Source: CAD feature listing. Evaluate the final solid. Frame: model axes, mm. Give positions to 0.01 mm unless a question says otherwise; leave off trailing zeros. Write each loop counter-clockwise with the first axis right and the second up, starting at its lowest first coordinate (ties: lowest second). Pieces come first, ordered by that corner, then holes. Notation, with made-up numbers: (83.5, -5.75) - (122.5, -5.75) arc R14 ccw to (122.5, 1.25) - close; hole circle Ø1 at (22.5, 12.5). An arc over 180 degrees is marked (long way). One line per question, with ' | ' between items. Start each with the question number.
(1) Section C-C, the plane x = 8. Return loops of the section in (y, z).
(2) Section A-A, the plane x = 16.5. Return loops of the section in (y, z).
(3) Section B-B, the plane y = 18.5. Return loops of the section in (x, z), plus the area to 3 significant figures.
(4) Ray query, line 1 (Z direction, x = -25, y = 0.5). Return the intervals inside material, ascending. Write a range as [from, to].
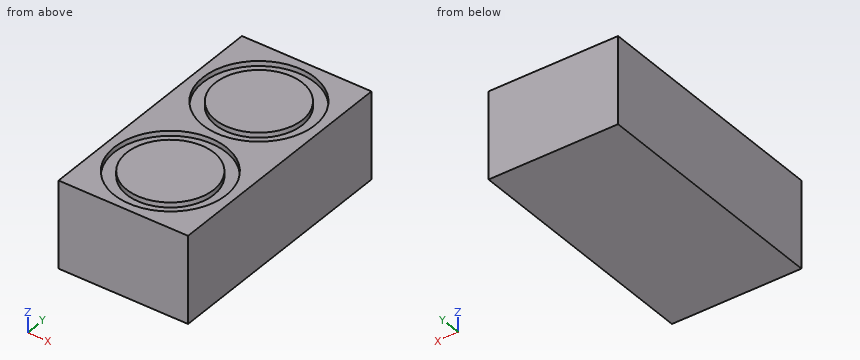
```python
from build123d import *

# Parameters (mm, degrees)
SKETCH_1_W          = 52
SKETCH_1_H          = 100
EXTRUDE_1_DEPTH     = 35
SKETCH_2_R          = 22.5
SKETCH_2_R_2        = 17.5
CUT_EXTRUDE_1_DEPTH = 2


with BuildPart() as part:
    # 草圖1 → 填料-伸長1 (new body)
    with BuildSketch(Plane.XY):
        with Locations((-4.941582483, -21.722113503)):
            Rectangle(SKETCH_1_W, SKETCH_1_H)
    extrude(amount=EXTRUDE_1_DEPTH)

    # 草圖2 → 除料-伸長1 (cut)
    # profile 1 of 2: a face of its own
    with BuildSketch(Plane.XY.offset(35)):
        with Locations((-4.941582483, 2.224790527)):
            Circle(SKETCH_2_R)
        with Locations((-4.941582483, 2.224790527)):
            Circle(SKETCH_2_R_2, mode=Mode.SUBTRACT)
    # profile 2 of 2: a face of its own
    with BuildSketch(Plane.XY.offset(35)):
        with Locations((-4.941582483, -46.083085038)):
            Circle(SKETCH_2_R)
        with Locations((-4.941582483, -46.083085038)):
            Circle(SKETCH_2_R_2, mode=Mode.SUBTRACT)
    extrude(amount=-CUT_EXTRUDE_1_DEPTH, mode=Mode.SUBTRACT)


solid = part.part
```
Check sheet entries:
1) outline: (-71.72, 0) - (28.28, 0) - (28.28, 35) - (20.63, 35) - (20.63, 33) - (14, 33) - (14, 35) - (-9.56, 35) - (-9.56, 33) - (-16.18, 33) - (-16.18, 35) - (-27.68, 35) - (-27.68, 33) - (-34.3, 33) - (-34.3, 35) - (-57.86, 35) - (-57.86, 33) - (-64.49, 33) - (-64.49, 35) - (-71.72, 35) - close
2) outline: (-71.72, 0) - (28.28, 0) - (28.28, 35) - (9.04, 35) - (9.04, 33) - (-4.59, 33) - (-4.59, 35) - (-39.26, 35) - (-39.26, 33) - (-52.9, 33) - (-52.9, 35) - (-71.72, 35) - close
3) outline: (-30.94, 0) - (21.06, 0) - (21.06, 35) - (10.59, 35) - (10.59, 33) - (1.49, 33) - (1.49, 35) - (-11.37, 35) - (-11.37, 33) - (-20.48, 33) - (-20.48, 35) - (-30.94, 35) - close | area: 1,780 mm²
4) line 1: [0, 33]
